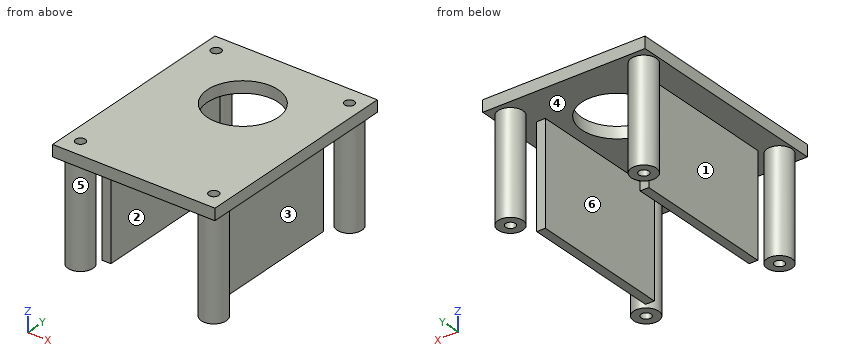
Solid Edge part; units mm, degrees
sketch "Sketch1" plane through (0, 0, -5) normal (0, 0, 1) x (1, 0, 0)
  line L0 (-28, -49) -> (28, -49)
  line L1 (28, -49) -> (28, 24)
  line L2 (28, 24) -> (-28, 24)
  line L3 (-28, 24) -> (-28, -49)
  circle A0 centre (0, 0) radius 12.2
  circle A1 centre (-23, -43) radius 1.7
  circle A2 centre (23, -43) radius 1.7
  circle A3 centre (-23, 18) radius 1.7
  circle A4 centre (23, 18) radius 1.7
extrude "ExtrudedProtrusion_1" add sketch "Sketch1" along normal blind 4
sketch "Sketch2" plane through (0, 0, -40) normal (0, 0, 1) x (1, 0, 0)
  circle A0 centre (-23, -43) radius 4.3
  circle A1 centre (-23, -43) radius 1.7
extrude "ExtrudedProtrusion_2" add sketch "Sketch2" along normal blind 35
sketch "Sketch3" plane through (0, 0, -40) normal (0, 0, 1) x (1, 0, 0)
  circle A0 centre (23, -43) radius 4.3
  circle A1 centre (23, -43) radius 1.7
extrude "ExtrudedProtrusion_3" add sketch "Sketch3" along normal blind 35
sketch "Sketch4" plane through (0, 0, -40) normal (0, 0, 1) x (1, 0, 0)
  circle A0 centre (-23, 18) radius 4.3
  circle A1 centre (-23, 18) radius 1.7
extrude "ExtrudedProtrusion_4" add sketch "Sketch4" along normal blind 35
sketch "Sketch5" plane through (0, 0, -40) normal (0, 0, 1) x (1, 0, 0)
  circle A0 centre (23, 18) radius 4.3
  circle A1 centre (23, 18) radius 1.7
extrude "ExtrudedProtrusion_5" add sketch "Sketch5" along normal blind 35
sketch "Sketch6" plane through (0, 0, -40) normal (0, 0, 1) x (1, 0, 0)
  line L0 (-19.35, -38) -> (-16.35, -38)
  line L1 (-16.35, -38) -> (-16.35, 11)
  line L2 (-16.35, 11) -> (-19.35, 11)
  line L3 (-19.35, 11) -> (-19.35, -38)
extrude "ExtrudedProtrusion_6" add sketch "Sketch6" along normal blind 35
sketch "Sketch7" plane through (0, 0, -40) normal (0, 0, 1) x (1, 0, 0)
  line L0 (16.35, -38) -> (19.35, -38)
  line L1 (19.35, -38) -> (19.35, 11)
  line L2 (19.35, 11) -> (16.35, 11)
  line L3 (16.35, 11) -> (16.35, -38)
extrude "ExtrudedProtrusion_7" add sketch "Sketch7" along normal blind 35
Here's how the part is built. I have some questions about the finished solid (model axes, mm). Face numbers are marked on the shaded views. A direction names the side the tool comes from. Round coordinates to 2 decimals unless told otherwise and drop trailing zeros. Write each loop counter-clockwise with the first axis right and the second up, starting at its lowest first coordinate (ties: lowest second). Pieces come first, ordered by that corner, then holes.
1. Suppose I cut it at B-B (x = 23). List the corners of the cut face in (y, z) for me, and give its area (3 significant figures).
2. Suppose I cut it at D-D (y = 0). List the corners of the cut face in (x, z) for me, and give its area (3 significant figures).
3. Suppose I cut it at C-C (y = 18). List the corners of the cut face in (x, z) for me, and give its area (3 significant figures).
4. Will these pins go through, and if not, where does the flat tip stop? pin 1 Ø14.5 at (x, y) = (0, 0) entering from +Z; pin 2 Ø17.5 at (y, z) = (-5.5, -31) entering from -X; pin 3 Ø4 at (x, z) = (-14.5, -16) entering from +Y; pin 4 Ø3.5 at (x, z) = (18, -14.5) entering from -Y.
5. I need wall thicknesses on L1, parallel to Y at x = -23, z = -20; L2, parallel to X at y = 8.5, z = -34; L3, parallel to X at y = 17.5, z = -35. Which ranges of each line are inside material? Lowest first, please.
6. Suppose I cut it at A-A (z = -32). State how many separate pieces and enclosed holes the cut face has, and give its area (3 significant figures).
7. If we mould it in two halves opening along Y, with no side actions, what happens to the marked faces 5 and 6? For each: released by +Y, released by -Y, zero draft, split by the parting line, or undercut.
8. For the marked faces 1, 2, 3 and 4, which set-ups out of +Z, -Z, +X, -X, +Y, -Y let a thin tool reach every point of the face, with its end or its side?
Answer sheet:
1. outline: (-49, -5) - (-47.3, -5) - (-47.3, -40) - (-44.7, -40) - (-44.7, -1) - (-49, -1) - close; (-41.3, -40) - (-38.7, -40) - (-38.7, -5) - (13.7, -5) - (13.7, -40) - (16.3, -40) - (16.3, -1) - (-41.3, -1) - close; (19.7, -40) - (22.3, -40) - (22.3, -5) - (24, -5) - (24, -1) - (19.7, -1) - close
1. area: 629 mm2
2. outline: (-28, -5) - (-19.35, -5) - (-19.35, -40) - (-16.35, -40) - (-16.35, -5) - (-12.2, -5) - (-12.2, -1) - (-28, -1) - close; (12.2, -5) - (16.35, -5) - (16.35, -40) - (19.35, -40) - (19.35, -5) - (28, -5) - (28, -1) - (12.2, -1) - close
2. area: 336 mm2
3. outline: (-28, -5) - (-27.3, -5) - (-27.3, -40) - (-24.7, -40) - (-24.7, -1) - (-28, -1) - close; (-21.3, -40) - (-18.7, -40) - (-18.7, -5) - (18.7, -5) - (18.7, -40) - (21.3, -40) - (21.3, -1) - (-21.3, -1) - close; (24.7, -40) - (27.3, -40) - (27.3, -5) - (28, -5) - (28, -1) - (24.7, -1) - close
3. area: 561 mm2
4. pin 1: passes through
4. pin 2: stops at x = -19.35
4. pin 3: stops at y = 11
4. pin 4: stops at y = -45.82
5. L1: y = -47.3 to -44.7, -41.3 to -38.7, 13.7 to 16.3, 19.7 to 22.3
5. L2: x = -19.35 to -16.35, 16.35 to 19.35
5. L3: x = -27.27 to -24.62, -21.38 to -18.73, 18.73 to 21.38, 24.62 to 27.27
6. separate pieces: 6
6. enclosed holes: 4
6. area: 490 mm2
7. face 5: undercut
7. face 6: zero draft
8. face 1: -Z, -X
8. face 2: -Z, +Y, -Y
8. face 3: -Z, +X
8. face 4: -Z
